from build123d import *

# Parameters (mm, degrees)
BOSS_EXTRUDE1_DEPTH                             = 17.5
SKETCH2_R                                       = 1.5
CUT_EXTRUDE1_DEPTH                              = 4.5
CSK_FOR_M3_OVAL_HEAD_MACHINE_SCREW1_D           = 3.4
CSK_FOR_M3_OVAL_HEAD_MACHINE_SCREW1_CSINK_D     = 6.3
CSK_FOR_M3_OVAL_HEAD_MACHINE_SCREW1_CSINK_ANGLE = 90
CUT_EXTRUDE2_DEPTH                              = 3.2


with BuildPart() as part:
    # Sketch1 → Boss-Extrude1 (new body)
    with BuildSketch(Plane(origin=(0, 0, 0), x_dir=(1, 0, 0), z_dir=(0, 1, 0))):
        Polygon((27.724299065, -2.579662371), (27.724299065, 43.920337629), (-26.775700935, 43.920337629), (-26.775700935, 230.920337629), (27.724299065, 230.920337629), (27.724299065, 277.420337629), (-26.775700935, 277.420337629), (-26.775700935, 289.920337629), (318.224299065, 289.920337629), (318.224299065, -15.079662371), (-26.775700935, -15.079662371), (-26.775700935, -2.579662371), align=None)
    extrude(amount=BOSS_EXTRUDE1_DEPTH)

    # Sketch2 → Cut-Extrude1 (cut)
    # profile 1 of 2: a face of its own
    with BuildSketch(Plane(origin=(0, 17.5, 0), x_dir=(1, 0, 0), z_dir=(0, 1, 0))):
        Polygon((5.694299065, 191.745337629), (-9.875700935, 191.745337629), (-9.875700935, 195.230337629), (-17.275700935, 195.230337629), (-17.275700935, 171.230337629), (-9.875700935, 171.230337629), (-9.875700935, 174.715337629), (5.694299065, 174.715337629), (5.694299065, 173.570337629), (13.094299065, 173.570337629), (13.094299065, 192.890337629), (5.694299065, 192.890337629), align=None)
        with Locations(Location((-13.275700935, 191.420337629, 0), (0, 0, 270))):
            Circle(SKETCH2_R, mode=Mode.SUBTRACT)
        with Locations(Location((-13.275700935, 175.040337629, 0), (0, 0, 270))):
            Circle(SKETCH2_R, mode=Mode.SUBTRACT)
        with Locations(Location((9.094299065, 189.050337629, 0), (0, 0, 270))):
            Circle(SKETCH2_R, mode=Mode.SUBTRACT)
        with Locations(Location((9.094299065, 177.410337629, 0), (0, 0, 270))):
            Circle(SKETCH2_R, mode=Mode.SUBTRACT)
    # profile 2 of 2: a face of its own
    with BuildSketch(Plane(origin=(0, 17.5, 0), x_dir=(1, 0, 0), z_dir=(0, 1, 0))):
        Polygon((5.694299065, 100.125337629), (-9.875700935, 100.125337629), (-9.875700935, 103.610337629), (-17.275700935, 103.610337629), (-17.275700935, 79.610337629), (-9.875700935, 79.610337629), (-9.875700935, 83.095337629), (5.694299065, 83.095337629), (5.694299065, 81.950337629), (13.094299065, 81.950337629), (13.094299065, 101.270337629), (5.694299065, 101.270337629), align=None)
        with Locations(Location((-13.275700935, 99.800337629, 0), (0, 0, 270))):
            Circle(SKETCH2_R, mode=Mode.SUBTRACT)
        with Locations(Location((-13.275700935, 83.420337629, 0), (0, 0, 270))):
            Circle(SKETCH2_R, mode=Mode.SUBTRACT)
        with Locations(Location((9.094299065, 97.430337629, 0), (0, 0, 270))):
            Circle(SKETCH2_R, mode=Mode.SUBTRACT)
        with Locations(Location((9.094299065, 85.790337629, 0), (0, 0, 270))):
            Circle(SKETCH2_R, mode=Mode.SUBTRACT)
    extrude(amount=-CUT_EXTRUDE1_DEPTH, mode=Mode.SUBTRACT)

    # CSK for M3 Oval Head Machine Screw1 (through all)
    with Locations(Plane(origin=(0, 0, 0), x_dir=(-1, 0, 0), z_dir=(0, -1, 0))):
        with Locations((13.275700935, 191.420337629), (13.275700935, 175.040337629), (-9.094299065, 177.410337629), (-9.094299065, 189.050337629), (13.275700935, 83.420337629), (13.275700935, 99.800337629), (-9.094299065, 97.430337629), (-9.094299065, 85.790337629)):
            CounterSinkHole(CSK_FOR_M3_OVAL_HEAD_MACHINE_SCREW1_D / 2, CSK_FOR_M3_OVAL_HEAD_MACHINE_SCREW1_CSINK_D / 2, counter_sink_angle=CSK_FOR_M3_OVAL_HEAD_MACHINE_SCREW1_CSINK_ANGLE)

    # Sketch7 → Cut-Extrude2 (cut)
    with BuildSketch(Plane(origin=(0, 17.5, 0), x_dir=(1, 0, 0), z_dir=(0, 1, 0))):
        Polygon((13.094299065, 183.230337629), (13.094299065, 216.730337629), (28.094299065, 224.230337629), (43.094299065, 224.230337629), (63.094299065, 207.230337629), (63.094299065, 149.730337629), (13.094299065, 149.730337629), align=None)
        Polygon((13.094299065, 91.610337629), (13.094299065, 125.110337629), (28.094299065, 132.610337629), (43.094299065, 132.610337629), (63.094299065, 115.610337629), (63.094299065, 58.110337629), (13.094299065, 58.110337629), align=None)
    extrude(amount=-CUT_EXTRUDE2_DEPTH, mode=Mode.SUBTRACT)


solid = part.part
The listing builds one solid part. Answer for the finished solid, in the listing's coordinates (mm). A direction names the side the tool comes from. Give positions to 0.01 mm unless a question says otherwise; leave off trailing zeros. Loops run counter-clockwise (first coordinate to the right, second up) from the corner with the lowest first, then second, coordinate; pieces in that order, holes last.
Item 1: A cutting plane is placed at B-B (z = -73). Give the vertices of the cut face in (x, y).
Derived:
outline: (-26.78, 0) - (318.22, 0) - (318.22, 17.5) - (63.09, 17.5) - (63.09, 14.3) - (13.09, 14.3) - (13.09, 17.5) - (-26.78, 17.5) - close
Item 2: A cutting plane is placed at A-A (x = 1). Give the vertices of the cut face in (y, z).
Derived:
outline: (0, -289.92) - (17.5, -289.92) - (17.5, -277.42) - (0, -277.42) - close; (0, -230.92) - (17.5, -230.92) - (17.5, -191.75) - (13, -191.75) - (13, -174.72) - (17.5, -174.72) - (17.5, -100.13) - (13, -100.13) - (13, -83.1) - (17.5, -83.1) - (17.5, -43.92) - (0, -43.92) - close; (0, 2.58) - (17.5, 2.58) - (17.5, 15.08) - (0, 15.08) - close
Item 3: Find the intervals of material crossed by line 1 along Z through (x, y) = (-2, 3.5); line 2 along X through (y, z) = (10.75, -263.5); line 3 along X through (y, z) = (11.25, -83), in increasing order.
Derived:
line 1: z = -289.92 to -277.42, -230.92 to -43.92, 2.58 to 15.08
line 2: x = 27.72 to 318.22
line 3: x = -26.78 to -14.92, -11.63 to 318.22
Item 4: Determine the mould class of faces 4 (the flat face through (318.224, 9, -140)), 5 (the flat face through (38, 14.3, -188)), 6 (the flat face through (143, 9, -289.92)) for opening direction Z: +Z half, -Z half, draft (parallel to the pull), parting line (faces both ways), or undercut.
Derived:
face 4: draft
face 5: undercut
face 6: -Z half
Item 5: This flat-tipped pin is pushed along its axis until it touches: pin 1 Ø4 at (x, z) = (-13.28, -191.42) entering from +Y. Where does it stop, or does it pass through?
Derived:
pin 1: stops at y = 13
Item 6: A cutting plane is placed at C-C (y = 9.5). Give the number of separate pieces and of enclosed holes in the cut face, then the cut area to 3 significant figures.
Derived:
separate pieces: 1
enclosed holes: 8
area: 100,000 mm2
Item 7: A cutting plane is placed at D-D (x = 49). Give the vertices of the cut face in (y, z).
Derived:
outline: (0, -289.92) - (17.5, -289.92) - (17.5, -219.21) - (14.3, -219.21) - (14.3, -149.73) - (17.5, -149.73) - (17.5, -127.59) - (14.3, -127.59) - (14.3, -58.11) - (17.5, -58.11) - (17.5, 15.08) - (0, 15.08) - close
Item 8: A tool of negligible diameter and unlimited length cuts with its end or side. For faces 1 (the flat face through (-26.776, 9, -136)), 2 (the flat face through (27.724, 9, -20)), 3 (the flat face through (38, 14.3, -96)), from which of +Z, -Z, +X, -X, +Y, -Y can it reach the whole face along a straight path? Write none if from no direction.
Derived:
face 1: +Z, -Z, -X, +Y, -Y
face 2: -X, +Y, -Y
face 3: +Y
